Read the model definition and answer for the solid it produces. Units are mm, in the model's axes. A direction names the side the tool comes from. Coordinates: 2 decimals unless noted, no trailing zeros. Write each loop counter-clockwise with the first axis right and the second up, starting at its lowest first coordinate (ties: lowest second). Pieces come first, ordered by that corner, then holes. Notation, with made-up numbers: (20.25, -14) -> (25.25, -14) arc R30 ccw to (25.25, 15) -> close; hole circle Ø5 at (63, 29). An arc over 180 degrees is marked (long way). Write item = value, one per line. Start each with the question number.
1) Section C-C (z = -23.5) is taken. Determine the outline of the cut face in (x, y), plus the area to 3 significant figures.
2) A tool of negligible diameter and unlimited length cuts with its end or side. For faces 5 (the face through (-6, 197, -12.7)), 6 (the face through (-139.675, -27, 0)), 7 (the face through (-146, 50.8, -6)), from which of +Z, -Z, +X, -X, +Y, -Y can it reach the whole face along a straight path? Write none if from no direction.
3) Flat-ended cylindrical pins translate along their axes: pin 1 Ø1.5 at (x, z) = (-112, -38.5) entering from -Y; pin 2 Ø14 at (x, y) = (-146, 198) entering from -Z; pin 3 Ø4 at (x, z) = (-8.5, -17) entering from +Y; pin 4 Ø4 at (y, z) = (196.85, -6.35) entering from +X. Find the tip coordinate at first contact, or state that the pin passes through.
4) For a pull along X with two mould halves and no side action, classify faces 1 (the face through (-152.4, 54, -10)), 2 (the face through (-12.7, 6, -26)), 3 (the face through (-6, 83, -12.7)), 4 (the face through (-38.1, 177, 3)) as released by +X, released by -X, zero draft, split by the parting line, or undercut.
5) Find the intervals of material crossed by line 1 along Z through (x, y) = (-8.25, 88.9) (3 decimals); line 2 along X through (y, z) = (56, -11); line 3 along Z through (x, y) = (-21, 186), in increasing order. Write a range as from..to.
6) Section B-B (y = 196.85) is taken. Determine the outline of the cut face in (x, z) (3 decimals).
7) Section D-D (y = -38) is taken. Determine the outline of the cut face in (x, z), plus the area to 3 significant figures.
8) Section A-A (x = -125) is taken. Determine the outline of the cut face in (y, z), plus the area to 3 significant figures.
from build123d import *

# Parameters (mm, degrees)
SKETCH1_W               = 152.4
SKETCH1_H               = 203.2
BOSS_EXTRUDE1_DEPTH     = 6.35
CUT_EXTRUDE1_DEPTH      = 255.079362602
CUT_EXTRUDE1_DEPTH_BACK = 255.079362602
SKETCH2_W               = 76.2
SKETCH2_H               = 50.8
SKETCH3_W               = 12.7
SKETCH3_H               = 12.7
SKETCH3_H_2             = 63.5
BOSS_EXTRUDE2_DEPTH     = 12.7
SKETCH4_R               = 3.175
CUT_EXTRUDE2_DEPTH      = 247.916220609
BOSS_EXTRUDE3_DEPTH     = 152.4
BOSS_EXTRUDE5_REACH     = 259.86
SKETCH11_W              = 12.72505143
SKETCH11_H              = 12.7
BOSS_EXTRUDE8_REACH     = 259.86
SKETCH13_W              = 12.7
SKETCH13_H              = 12.7


with BuildPart() as part:
    # Sketch1 → Boss-Extrude1 (new body)
    with BuildSketch(Plane.XY):
        with Locations((-76.2, 101.6)):
            Rectangle(SKETCH1_W, SKETCH1_H)
    extrude(amount=BOSS_EXTRUDE1_DEPTH)

    # Sketch2 → Cut-Extrude1 (cut, two sides: drawn at the far end of the back side and taken through both)
    with BuildSketch(Plane.XY.offset(6.35).offset(-CUT_EXTRUDE1_DEPTH_BACK)):
        with Locations((-76.2, 177.8)):
            Rectangle(SKETCH2_W, SKETCH2_H)
    extrude(amount=CUT_EXTRUDE1_DEPTH + CUT_EXTRUDE1_DEPTH_BACK, mode=Mode.SUBTRACT)

    # Sketch3 → Boss-Extrude2 (add)
    with BuildSketch(Plane(origin=(0, 0, 0), x_dir=(-1, 0, 0), z_dir=(0, 0, -1))):
        with Locations((146.05, 196.85)):
            Rectangle(SKETCH3_W, SKETCH3_H)
        with Locations((146.05, 82.55)):
            Rectangle(SKETCH3_W, SKETCH3_H_2)
    boss_extrude2 = extrude(amount=BOSS_EXTRUDE2_DEPTH)

    # Sketch4 → Cut-Extrude2 (cut, symmetric)
    with BuildSketch(Plane(origin=(-139.7, 0, 0), x_dir=(0, 0, -1), z_dir=(1, 0, 0))):
        with Locations((6.35, 196.85)):
            Circle(SKETCH4_R)
        with Locations((6.35, 101.6)):
            Circle(SKETCH4_R)
        with Locations((6.35, 88.9)):
            Circle(SKETCH4_R)
        with Locations((6.35, 76.2)):
            Circle(SKETCH4_R)
        with Locations((6.35, 63.5)):
            Circle(SKETCH4_R)
    cut_extrude2 = extrude(amount=CUT_EXTRUDE2_DEPTH, both=True, mode=Mode.SUBTRACT)



with BuildPart() as body_2:
    # Sketch6 → Boss-Extrude3 (new body)
    with BuildSketch(Plane(origin=(0, 0, 0), x_dir=(0, 0, -1), z_dir=(1, 0, 0))):
        Polygon((44.45, 0), (-6.35, -75.934955719), (-6.35, -71.366926193), (41.394017446, 0), align=None)
    extrude(amount=-BOSS_EXTRUDE3_DEPTH)


with BuildPart() as body_3:
    # Boss-Extrude5: up to this plane
    boss_extrude5_end = Plane(origin=(-243.760590519, 0, -41.394017446), z_dir=(0, 0.5560384374855327, 0.8311565773298358))
    # Sketch11 → Boss-Extrude5 (new, up to the surface)
    with BuildSketch(Plane(origin=(0, 0, 0), x_dir=(-1, 0, 0), z_dir=(0, -1, 0)), mode=Mode.PRIVATE) as boss_extrude5_sk1:
        with Locations((146.037474285, 0)):
            Rectangle(SKETCH11_W, SKETCH11_H)
    boss_extrude5_tool1 = split(extrude(boss_extrude5_sk1.sketch, amount=BOSS_EXTRUDE5_REACH, mode=Mode.PRIVATE), bisect_by=boss_extrude5_end, keep=Keep.BOTH, mode=Mode.PRIVATE)
    add(boss_extrude5_tool1.solids().sort_by_distance((-146.037474, 0, 0))[0])


with BuildPart() as part_1:
    add(part.part)

    add(body_2.part)  # Boss-Extrude8 merges body 2

    add(body_3.part)  # Boss-Extrude8 merges body 3
    # Boss-Extrude8: up to this plane
    boss_extrude8_end = Plane(origin=(-243.760590519, 0, -44.45), z_dir=(0, -0.5560384374855327, -0.8311565773298358))
    # Sketch13 → Boss-Extrude8 (add, up to the surface)
    with BuildSketch(Plane(origin=(0, 0, 0), x_dir=(-1, 0, 0), z_dir=(0, 0, -1)), mode=Mode.PRIVATE) as boss_extrude8_sk1:
        with Locations((146.05, 6.35)):
            Rectangle(SKETCH13_W, SKETCH13_H)
    boss_extrude8_tool1 = split(extrude(boss_extrude8_sk1.sketch, amount=BOSS_EXTRUDE8_REACH, mode=Mode.PRIVATE), bisect_by=boss_extrude8_end, keep=Keep.BOTH, mode=Mode.PRIVATE)
    boss_extrude8 = boss_extrude8_tool1.solids().sort_by_distance((-146.05, 6.35, 0))[0]
    add(boss_extrude8)

    # Mirror1: Boss-Extrude2, Cut-Extrude2, Boss-Extrude8 across plane
    add(boss_extrude2.mirror(Plane.ZY.offset(76.2)))
    add(cut_extrude2.mirror(Plane.ZY.offset(76.2)), mode=Mode.SUBTRACT)
    add(boss_extrude8.mirror(Plane.ZY.offset(76.2)))


solid = part_1.part
Answer key:
q1.outline = (-152.4, -31.32) -> (0, -31.32) -> (0, -26.75) -> (-152.4, -26.75) -> close; (-152.4, 0) -> (-139.7, 0) -> (-139.7, 12.7) -> (-152.4, 12.7) -> close; (-12.7, 0) -> (0, 0) -> (0, 12.7) -> (-12.7, 12.7) -> close
q1.area = 1,020 mm^2
q2.face_5 = -Z, +X, -X, +Y
q2.face_6 = +Z, +X
q2.face_7 = -Z, +X, -X
q3.pin_1 = -10.02
q3.pin_2 = -12.7
q3.pin_3 = 12.7
q3.pin_4 = through
q4.face_1 = released by -X
q4.face_2 = undercut
q4.face_3 = zero draft
q4.face_4 = undercut
q5.line_1 = -12.7..-9.525, -3.175..6.35
q5.line_2 = -152.4..-139.7, -12.7..0
q5.line_3 = 0..6.35
q6.outline = (-152.4, -12.7) -> (-139.7, -12.7) -> (-139.7, -9.525) -> (-152.4, -9.525) -> close; (-152.4, -3.175) -> (-139.7, -3.175) -> (-139.7, 0) -> (-114.3, 0) -> (-114.3, 6.35) -> (-152.4, 6.35) -> close; (-38.1, 0) -> (-12.7, 0) -> (-12.7, -3.175) -> (0, -3.175) -> (0, 6.35) -> (-38.1, 6.35) -> close; (-12.7, -12.7) -> (0, -12.7) -> (0, -9.525) -> (-12.7, -9.525) -> close
q7.outline = (-152.4, -19.03) -> (0, -19.03) -> (0, -15.97) -> (-152.4, -15.97) -> close; (-152.4, -6.35) -> (-139.67, -6.35) -> (-139.67, 6.35) -> (-152.4, 6.35) -> close
q7.area = 627 mm^2
q8.outline = (-75.93, 6.35) -> (0, -44.45) -> (0, -41.39) -> (-71.37, 6.35) -> close; (0, 0) -> (203.2, 0) -> (203.2, 6.35) -> (0, 6.35) -> close
q8.area = 1,520 mm^2
